from build123d import *

# Parameters (mm, degrees)
F1_DEPTH = 101.6
F2_R     = 3.69316
F3_R     = 1.98374
F4_R     = 1.8288
F5_DEPTH = 95.37192
F6_R     = 5.55625
F7_R     = 1.8288
F8_DEPTH = 1.70942


with BuildPart() as f1:
    # F0 (on Top) → F1 (new body)
    with BuildSketch(Plane.XY):
        Polygon((0, 13.09624), (0, 0), (-91.95308, 0), (-91.95308, 13.09624), (-93.6625, 13.09624), (-93.6625, -1.70942), (1.70942, -1.70942), (1.70942, 13.09624), align=None)
    extrude(amount=F1_DEPTH)

    # F2
    f2_edges = [f1.edges().sort_by_distance(p)[0] for p in [
        (1.70942, -1.70942, 50.8),
        (-93.6625, -1.70942, 50.8),
    ]]
    fillet(f2_edges, radius=F2_R)

    # F3
    f3_edges = [f1.edges().sort_by_distance(p)[0] for p in [
        (0, 0, 50.8),
        (-91.95308, 0, 50.8),
    ]]
    fillet(f3_edges, radius=F3_R)

    # F4 (on face) → F5 (cut, through all)
    with BuildSketch(Plane.YZ.offset(1.70942)):
        with Locations((7.53999, 96.04375)):
            Circle(F4_R)
        with Locations((7.53999, 5.55625)):
            Circle(F4_R)
    extrude(amount=-F5_DEPTH, mode=Mode.SUBTRACT)

    # F6
    f6_edges = [f1.edges().sort_by_distance(p)[0] for p in [
        (-92.80779, 13.09624, 101.6),
        (-92.80779, 13.09624, 0),
        (0.85471, 13.09624, 0),
        (0.85471, 13.09624, 101.6),
    ]]
    fillet(f6_edges, radius=F6_R)

    # F7 (on face) → F8 (cut, through all)
    with BuildSketch(Plane(origin=(0, 0, 0), x_dir=(-1, 0, 0), z_dir=(0, 1, 0))):
        with Locations((59.0904203, 44.1744082526)):
            Circle(F7_R)
        with Locations((45.97654, 57.4255917474)):
            Circle(F7_R)
        with Locations((32.8626597, 44.1744082526)):
            Circle(F7_R)
    extrude(amount=-F8_DEPTH, mode=Mode.SUBTRACT)


solid = f1.part
Check sheet for the modelled part. Datum: model origin and axes. Units: mm. A direction names the side the tool comes from. Give positions to 0.01 mm unless a question says otherwise; leave off trailing zeros. Write each loop counter-clockwise with the first axis right and the second up, starting at its lowest first coordinate (ties: lowest second). Pieces come first, ordered by that corner, then holes. Notation, with made-up numbers: M 58,38 L 64,38 A24 cw 64,58 Z; hole C 4,0.5 d5. An arc over 180 degrees is marked long. Use one line per item in the form item = value.
(1) Depth check by flat-ended pin: P1, Ø3, axis at x = -45.98, z = 57.43, coming from the +Y side; P2, Ø5, axis at y = 7.54, z = 96.04, coming from the -X side; P3, Ø1.5, axis at x = -13.5, z = 39.5, coming from the +Y side. Enter the tip coordinate at first touch or a pass-through.
Answer block:
P1 = through
P2 = -93.66
P3 = 0
(2) Draft check along Z on faces 1 (the cylindrical face through (0.843, 11.425, 1.584)), 2 (the cylindrical face through (0.87, 9.23, 4.86)), 3 (the cylindrical face through (0.84, 11.51, 99.93)). Enter one of: pulls with the +Z half, pulls with the -Z half, needs draft (parallel to the pull), parting line crosses it, or undercut.
Answer block:
face_1 = pulls with the -Z half
face_2 = undercut
face_3 = pulls with the +Z half
(3) Tool access check on faces 4 (the flat face through (0, 8, 50)), 5 (the cylindrical face through (-92.82, 11.51, 99.93)). Record the directions out of +Z, -Z, +X, -X, +Y, -Y that give a thin tool (end or side, any length) a straight path to the whole face; none if there is none.
Answer block:
face_4 = +Z, -Z, +Y
face_5 = +Z, +X, -X, +Y
(4) Section check B-B on x = -73. Record the boundary of the cut face in (y, z), plus the area to 3 significant figures.
Answer block:
outline = M -1.71,0 L 0,0 L 0,101.6 L -1.71,101.6 Z
area = 174 mm2
(5) Section check A-A on z = 75.5. Record the boundary of the cut face in (x, y).
Answer block:
outline = M -93.66,1.98 A3.69 ccw -89.97,-1.71 L -1.98,-1.71 A3.69 ccw 1.71,1.98 L 1.71,13.1 L 0,13.1 L 0,1.98 A1.98 cw -1.98,0 L -89.97,0 A1.98 cw -91.95,1.98 L -91.95,13.1 L -93.66,13.1 Z
(6) Material ranges on line 1 along X through (y, z) = (7, 24); line 2 along Y through (x, z) = (-6, 23); line 3 along X through (y, z) = (-0.75, 41), recorded low to high.
Answer block:
line_1 = -93.66 to -91.95, 0 to 1.71
line_2 = -1.71 to 0
line_3 = -92.45 to 0.5
